Autodesk Fusion 360 part; units mm, degrees
sketch "Sketch1" plane through (0, 0, 0) normal (0, 0, 1) x (1, 0, 0)
  circle A0 centre (0, 0) radius 23.5
  dimension "d1" = 47
extrude "Extrude1" add sketch "Sketch1" along normal blind 3 makes body 1
fillet "Fillet1" radius 3 1 edges at (-21.9097, -8.498, 0) on bodies 1
sketch "Sketch2" plane through (0, 0, 3) normal (0, 0, 1) x (1, 0, 0)
  circle A0 centre (0, 0) radius 23.5
  circle A1 centre (0, 0) radius 14
  dimension "d5" = 28
extrude "Extrude2" add sketch "Sketch2" along normal blind 13 contours A1 bodies 1
sketch "Sketch3" plane through (0, 0, 16) normal (0, 0, 1) x (1, 0, 0)
  circle A0 centre (0, 0) radius 14
  circle A1 centre (0, 0) radius 20
  dimension "d8" = 40
extrude "Extrude3" add sketch "Sketch3" along normal blind 1 separate body makes body 2
fillet "Fillet2" radius 1 1 edges at (-18.6465, -7.2323, 17) on bodies 2
sketch "Sketch4" plane through (0, 0, 16) normal (0, 0, 1) x (1, 0, 0)
  circle A0 centre (0, 0) radius 14
  circle A1 centre (0, 0) radius 20.5
extrude "Extrude4" add sketch "Sketch4" along normal blind 6 contours A0 bodies 1 2
sketch "Sketch5" plane through (0, 0, 22) normal (0, 0, 1) x (1, 0, 0)
  circle A0 centre (0, 0) radius 14
  circle A1 centre (0, 0) radius 20.5
  circle A2 centre (0, 0) radius 18.5
  dimension "d14" = 37
extrude "Extrude5" add sketch "Sketch5" along normal blind 0.9 separate body contours A1 | A2 makes body 3
fillet "Fillet3" radius 0.9 1 edges at (-19.1127, -7.4131, 22.9) on bodies 3
extrude "Extrude6" add 1 faces at (3.6071, -3.6485, 22) along direction (0, 0, 1) blind 5 on bodies 1 bodies 1 3
sketch "Sketch6" plane through (0, 0, 27) normal (0, 0, 1) x (1, 0, 0)
  circle A0 centre (0, 0) radius 14
  circle A1 centre (0, 0) radius 20.5
  circle A2 centre (0, 0) radius 17
  dimension "d20" = 34
extrude "Extrude7" add sketch "Sketch6" along normal blind 0.7 separate body contours A1 | A2 makes body 4
fillet "Fillet4" radius 0.7 1 edges at (-19.1127, -7.4131, 27.7) on bodies 4
extrude "Extrude8" add 1 faces at (3.6071, -3.6485, 27) along direction (0, 0, 1) blind 6 on bodies 1 bodies 1 4
sketch "Sketch7" plane through (0, 0, 33) normal (0, 0, 1) x (1, 0, 0)
  circle A0 centre (0, 0) radius 14
  circle A1 centre (0, 0) radius 20.5
  circle A2 centre (0, 0) radius 11.75
  dimension "d26" = 23.5
extrude "Extrude9" cut sketch "Sketch7" against normal blind 30 contours A2 bodies 1
equation "d24 = 30 mm - 13 mm - 6 mm - 5 mm"
Check sheet for the modelled part. Datum: model origin and axes. Units: mm. A direction names the side the tool comes from. Coordinates: 2 decimals unless noted, no trailing zeros. Order: outer loops, then holes, each group sorted by start corner. A loop starts at its lowest first (then second) coordinate and runs counter-clockwise, first axis right, second up. Notation, with made-up numbers: (-9.75, 79) -> (25.25, 79) arc R24 ccw to (25.25, 103) -> close; hole circle Ø8 at (82, 75.5). An arc over 180 degrees is marked (long way). Write item = value, one per line. Start each with the question number.
1) Material ranges on L1, parallel to Z at x = 15, y = -7.5; L2, parallel to Y at x = 0, z = 23.75; L3, parallel to Z at x = 3, y = 7, recorded low to high.
2) Cross-section at D-D (z = 2). Enter the section's corners in (x, y), then the cut area to 3 significant figures.
3) Access from +Z, -Z, +X, -X, +Y, -Y to the whole of each face (thin tool, end or side, straight path). Record for faces 4 (the flat face through (10.1, -10.1, 3)), 5 (the cylindrical face through (12.932, 5.362, 30.313)), 6 (the flat face through (0, 0, 0)).
4) Mould release check, pull along Y, two halves, no side actions. Record for faces 1 (the cylindrical face through (11.207, 3.529, 18.21)), 2 (the flat face through (-4.8, -13.4, 27)), 3 (the cylindrical face through (12.932, 5.362, 9.409)): +Y half, -Y half, draft (parallel to the pull), parting line (faces both ways), or undercut.
5) Cross-section at B-B (y = 17). State how many separate pieces and enclosed holes the cut face has, then the cut area to 3 significant figures.
6) Go/stop test with flat-tipped pins: P1, Ø12, axis at x = -12, z = 13.5, coming from the -Y side; P2, Ø19, axis at x = 0, y = 0, coming from the +Z side; P3, Ø5, axis at x = 3.5, z = 20.5, coming from the +Y side. Record where each tip stops, or that it passes through.
7) Cross-section at A-A (z = 5.5). Enter the section's corners in (x, y).
Ans:
q1.L1 = 0 to 3, 16 to 17, 22 to 22.9, 27 to 27.7
q1.L2 = -14 to -11.75, 11.75 to 14
q1.L3 = 0 to 3
q2.outline = circle Ø46.66 at (0, 0)
q2.area = 1,710 mm²
q3.face_4 = none
q3.face_5 = +Z
q3.face_6 = -Z, +X, -X, +Y, -Y
q4.face_1 = undercut
q4.face_2 = draft
q4.face_3 = parting line
q5.separate_pieces = 4
q5.enclosed_holes = 0
q5.area = 147 mm²
q6.P1 = -18.9
q6.P2 = 3
q6.P3 = 20.45
q7.outline = circle Ø28 at (0, 0); hole circle Ø23.5 at (0, 0)
